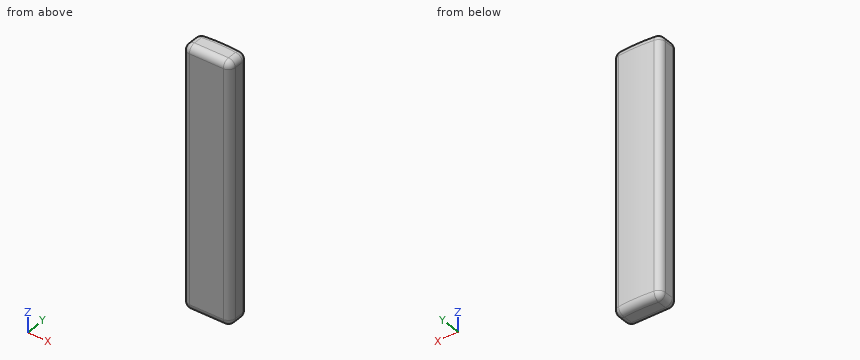
```python
from build123d import *

# Parameters (mm, degrees)
SKETCH1_W           = 7
SKETCH1_H           = 3.5
BOSS_EXTRUDE1_DEPTH = 38
SKETCH2_R           = 29
SKETCH2_R_2         = 24
CUT_EXTRUDE1_DEPTH  = 39.200948941
FILLET1_R           = 1


with BuildPart() as part:
    # Sketch1 → Boss-Extrude1 (new body)
    with BuildSketch(Plane.XY):
        Rectangle(SKETCH1_W, SKETCH1_H)
    extrude(amount=BOSS_EXTRUDE1_DEPTH)

    # Sketch2 → Cut-Extrude1 (cut, through all)
    with BuildSketch(Plane.XY.offset(38)):
        with Locations((0, -22.25)):
            Circle(SKETCH2_R)
        with Locations((0, -22.25)):
            Circle(SKETCH2_R_2, mode=Mode.SUBTRACT)
    extrude(amount=-CUT_EXTRUDE1_DEPTH, mode=Mode.SUBTRACT)

    # Fillet1
    fillet1_edges = [part.edges().sort_by_distance(p)[0] for p in [
        (0, -1.75, 38),
        (-3.5, -0.128289929, 0),
        (0, 1.75, 0),
        (-3.5, -0.128289929, 38),
        (0, 1.75, 38),
        (3.5, 1.493420141, 19),
        (-3.5, 1.493420141, 19),
        (3.5, -0.128289929, 38),
        (0, -1.75, 0),
        (3.5, -0.128289929, 0),
        (3.5, -1.75, 19),
        (-3.5, -1.75, 19),
    ]]
    fillet(fillet1_edges, radius=FILLET1_R)


solid = part.part
```
Could you check a few things on this model? Use its own coordinates, in mm. Coordinates: 2 decimals unless noted, no trailing zeros. Loops run counter-clockwise (first coordinate to the right, second up) from the corner with the lowest first, then second, coordinate; pieces in that order, holes last. Notation, with made-up numbers: M -30.5,73 L 17.5,73 A17 cw 17.5,84 Z; hole C 76,-19.75 d5. An arc over 180 degrees is marked long. Put each result on its own line as item: value. Start each with the question number.
(1) I need wall thicknesses on line 1 (Y direction, x = -0.5, z = 26); line 2 (X direction, y = -0.8, z = 11); line 3 (Z direction, x = 0.75, y = -0.95). Which ranges of each line are inside material? Lowest first, please. Write a range as from..to.
(2) Suppose I cut it at A-A on z = 25.5. Please give me the cut outline in (x, y).
(3) Suppose I cut it at B-B on x = 3. Please give me the cut outline in (y, z), then the cut area to 3 significant figures.
Solutions:
1. line 1: y = -1.75..1.74
1. line 2: x = -3.5..3.5
1. line 3: z = 0.02..37.98
2. outline: M -3.5,-0.75 A1 ccw -2.5,-1.75 L 2.5,-1.75 A1 ccw 3.5,-0.75 L 3.5,0.61 A1 ccw 2.61,1.61 A24 ccw -2.61,1.61 A1 ccw -3.5,0.61 Z
3. outline: M -1.62,1 A0.87 ccw -0.75,0.13 L 0.61,0.13 A0.87 ccw 1.48,1 L 1.48,37 A0.87 ccw 0.61,37.87 L -0.75,37.87 A0.87 ccw -1.62,37 Z
3. area: 116 mm2
